Read the model definition and answer for the solid it produces. Units are mm, in the model's axes. A direction names the side the tool comes from. Coordinates: 2 decimals unless noted, no trailing zeros. Order: outer loops, then holes, each group sorted by start corner. A loop starts at its lowest first (then second) coordinate and runs counter-clockwise, first axis right, second up. Notation, with made-up numbers: (20, 81.5) -> (72, 81.5) arc R31 cw to (72, 109.5) -> close; hole circle Ø2 at (35, 36.25). An arc over 180 degrees is marked (long way). Answer as a JSON object with one key per item and string values. Group by question number.
1) Section A-A on x = 9 is taken. Determine the outline of the cut face in (y, z), and give its area (3 significant figures).
2) Section B-B on y = 109.5 is taken. Determine the outline of the cut face in (x, z), and give its area (3 significant figures).
3) A tool of negligible diameter and unlimited length cuts with its end or side. For faces 4 (the flat face through (62, 295, 2)), 5 (the flat face through (62, 300, 2)), from which of +Z, -Z, +X, -X, +Y, -Y can it reach the whole face along a straight path? Write none if from no direction.
4) Consider L1, parallel to X at y = 106, z = 3.15; L2, parallel to Y at x = 93.5, z = 4.65. Determine where each line is inside the solid, lowest interval first.
5) Determine the mould class of faces 1 (the flat face through (126, 148, 2)), 2 (the flat face through (64, 5, 2)), 3 (the flat face through (62, 0, 2)) for opening direction X: released by +X, released by -X, zero draft, split by the parting line, or undercut.
from build123d import *

# Parameters (mm, degrees)
F0_W     = 126
F0_H     = 300
F1_DEPTH = 5


with BuildPart() as f1:
    # F0 (on Top) → F1 (new body)
    with BuildSketch(Plane.XY):
        with Locations((63, 150)):
            Rectangle(F0_W, F0_H)
        Polygon((34, 5), (5, 5), (5, 34), (5, 63), (5, 92), (5, 121), (5, 150), (5, 179), (5, 208), (5, 237), (5, 266), (5, 295), (34, 295), (63, 295), (92, 295), (121, 295), (121, 266), (121, 237), (121, 208), (120.960728, 208), (121, 179), (121, 150), (121, 121), (121, 92), (121, 63), (121, 34), (121, 5), (92, 5), (63, 5), align=None, mode=Mode.SUBTRACT)
    extrude(amount=F1_DEPTH)


solid = f1.part
Worked answers:
{
 "1": {"outline": "(0, 0) -> (5, 0) -> (5, 5) -> (0, 5) -> close; (295, 0) -> (300, 0) -> (300, 5) -> (295, 5) -> close", "area": "50.0 mm²"},
 "2": {"outline": "(0, 0) -> (5, 0) -> (5, 5) -> (0, 5) -> close; (121, 0) -> (126, 0) -> (126, 5) -> (121, 5) -> close", "area": "50.0 mm²"},
 "3": {"face 4": "+Z, -Z", "face 5": "+Z, -Z, +X, -X, +Y"},
 "4": {"L1": "x = 0 to 5, 121 to 126", "L2": "y = 0 to 5, 295 to 300"},
 "5": {"face 1": "released by +X", "face 2": "undercut", "face 3": "zero draft"}
}
